Geometry check sheet. Reference: drawing and pictorial views, mm from the part's lowest x, y, z. A direction names the side the tool comes from. Round coordinates to 2 decimals unless told otherwise and drop trailing zeros. Order: outer loops, then holes, each group sorted by start corner. A loop starts at its lowest first (then second) coordinate and runs counter-clockwise, first axis right, second up. Notation, with made-up numbers: M -8.75,71.5 L 11.25,71.5 A19 cw 11.25,97.5 Z; hole C 34,38.5 d6. An arc over 180 degrees is marked long. Answer as a JSON object with one key per item and string values. Group by question number.
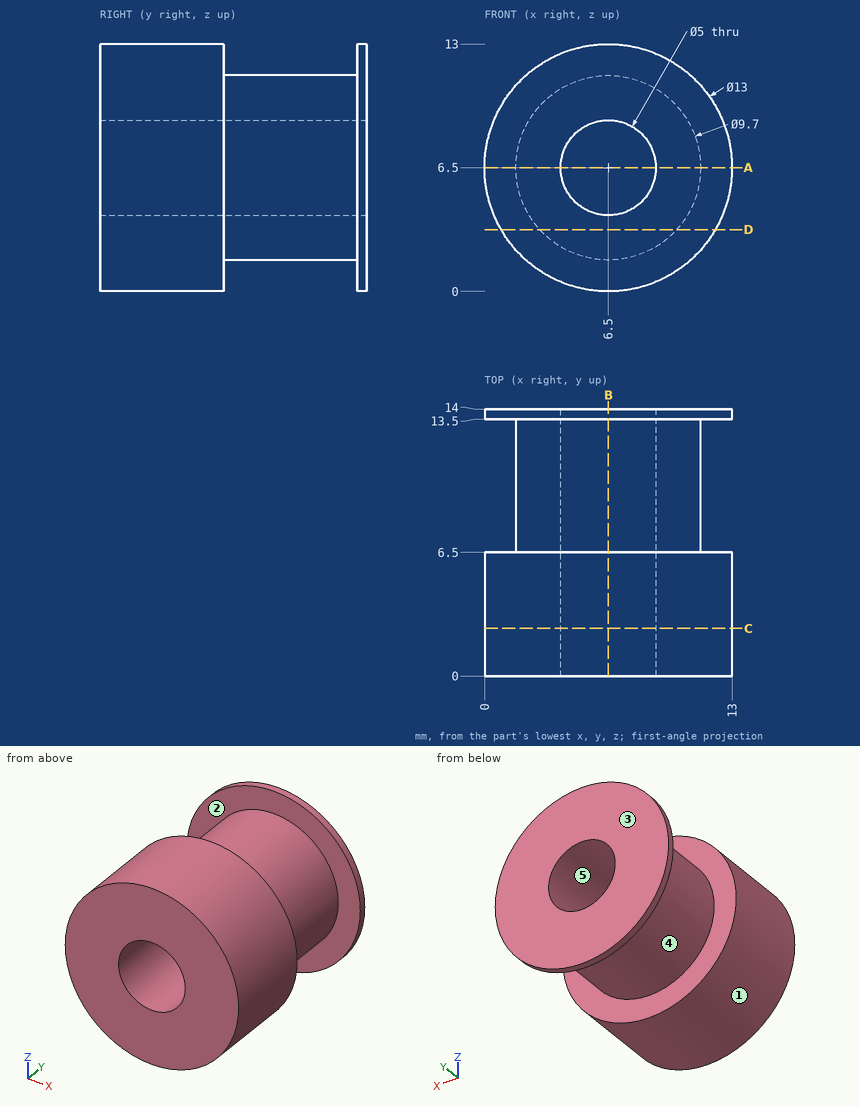
Q1. Release check for a two-part mould opening along X. For the marked faces 3, 4 and 5 record: released by +X, released by -X, zero draft, split by the parting line, or undercut.
Q2. Gauge pin test, flat ends, axial feed: pin 1 Ø4 at (x, z) = (3, 2) entering from -Y; pin 2 Ø1.5 at (y, z) = (2.5, 4.5) entering from -X; pin 3 Ø1 at (y, z) = (1.5, 7.5) entering from +X; pin 4 Ø1 at (x, y) = (9, 10.5) entering from +Z. Record the tip position at first contact, or that the pin passes through.
Q3. Cross-section at B-B, the plane x = 6.5. Record the cut outline in (y, z).
Q4. Thickness scan on line 1 (X direction, y = 11, z = 6.5); line 2 (Y direction, x = 11.5, z = 10). Record the ranges inside material, lowest first. Write a range as from..to.
Q5. Cross-section at D-D, the plane z = 3.25. Record the cut outline in (x, y).
Q6. Cross-section at A-A, the plane z = 6.5. Record the cut outline in (x, y), then the cut area to 3 significant figures.
Q7. Tool access check on the marked faces 1 and 2. Record the directions out of +Z, -Z, +X, -X, +Y, -Y that give a thin tool (end or side, any length) a straight path to the whole face; none if there is none.
Q8. Cross-section at C-C, the plane y = 2.5. Record the cut outline in (x, z).
Conclusion:
{
 "1": {"face 3": "zero draft", "face 4": "split by the parting line", "face 5": "undercut"},
 "2": {"pin 1": "y = 0", "pin 2": "x = 0.12", "pin 3": "x = 12.98", "pin 4": "z = 10.92"},
 "3": {"outline": "M 0,0 L 6.5,0 L 6.5,1.65 L 13.5,1.65 L 13.5,0 L 14,0 L 14,4 L 0,4 Z; M 0,9 L 14,9 L 14,13 L 13.5,13 L 13.5,11.35 L 6.5,11.35 L 6.5,13 L 0,13 Z"},
 "4": {"line 1": "1.65..4, 9..11.35", "line 2": "0..6.5, 13.5..14"},
 "5": {"outline": "M 0.87,0 L 12.13,0 L 12.13,6.5 L 10.1,6.5 L 10.1,13.5 L 12.13,13.5 L 12.13,14 L 0.87,14 L 0.87,13.5 L 2.9,13.5 L 2.9,6.5 L 0.87,6.5 Z"},
 "6": {"outline": "M 0,0 L 4,0 L 4,14 L 0,14 L 0,13.5 L 1.65,13.5 L 1.65,6.5 L 0,6.5 Z; M 9,0 L 13,0 L 13,6.5 L 11.35,6.5 L 11.35,13.5 L 13,13.5 L 13,14 L 9,14 Z", "area": "88.9 mm2"},
 "7": {"face 1": "+Y, -Y", "face 2": "none"},
 "8": {"outline": "C 6.5,6.5 d13; hole C 6.5,6.5 d5"}
}
